Autodesk Inventor part; units mm, degrees
ref_plane "YZ Plane" through (0, 0, 0) normal (1, 0, 0) x (0, 1, 0)
ref_plane "XZ Plane" through (0, 0, 0) normal (0, 1, 0) x (-1, 0, 0)
ref_plane "XY Plane" through (0, 0, 0) normal (0, 0, 1) x (1, 0, 0)
sketch "Skin Scheme" plane through (0, 0, 0) normal (0, 1, 0) x (-1, 0, 0)
  line L0 (464, -84.5) -> (-464, -84.5)
  line L1 (-464, -84.5) -> (-464, 84.5)
  line L2 (-464, 84.5) -> (464, 84.5)
  line L3 (464, 84.5) -> (464, -84.5)
  circle A0 centre (342, -62.5) radius 5
  circle A1 centre (306, -62.5) radius 5
  circle A2 centre (270, -62.5) radius 5
  circle A3 centre (234, -62.5) radius 5
  circle A4 centre (198, -62.5) radius 5
  circle A5 centre (162, -62.5) radius 5
  circle A6 centre (126, -62.5) radius 5
  circle A7 centre (90, -62.5) radius 5
  circle A8 centre (54, -62.5) radius 5
  circle A9 centre (18, -62.5) radius 5
  circle A10 centre (-18, -62.5) radius 5
  circle A11 centre (-54, -62.5) radius 5
  circle A12 centre (-90, -62.5) radius 5
  circle A13 centre (-126, -62.5) radius 5
  circle A14 centre (-162, -62.5) radius 5
  circle A15 centre (-198, -62.5) radius 5
  circle A16 centre (-234, -62.5) radius 5
  circle A17 centre (-270, -62.5) radius 5
  circle A18 centre (342, 62.5) radius 5
  circle A19 centre (306, 62.5) radius 5
  circle A20 centre (270, 62.5) radius 5
  circle A21 centre (234, 62.5) radius 5
  circle A22 centre (198, 62.5) radius 5
  circle A23 centre (162, 62.5) radius 5
  circle A24 centre (126, 62.5) radius 5
  circle A25 centre (90, 62.5) radius 5
  circle A26 centre (54, 62.5) radius 5
  circle A27 centre (18, 62.5) radius 5
  circle A28 centre (-18, 62.5) radius 5
  circle A29 centre (-54, 62.5) radius 5
  circle A30 centre (-90, 62.5) radius 5
  circle A31 centre (-126, 62.5) radius 5
  circle A32 centre (-162, 62.5) radius 5
  circle A33 centre (-198, 62.5) radius 5
  circle A34 centre (-234, 62.5) radius 5
  circle A35 centre (-270, 62.5) radius 5
  circle A36 centre (-306, -62.5) radius 5
  circle A37 centre (-306, 62.5) radius 5
  circle A38 centre (-342, -62.5) radius 5
  circle A39 centre (-342, 62.5) radius 5
  point P0 (0, 0)
  dimension "d0" = 928
  dimension "d1" = 464
  dimension "d2" = 169
  dimension "d3" = 84.5
  dimension "d4" = 10
  dimension "d5" = 122
  dimension "d6" = 22
  dimension "d9" = 36
  dimension "d12" = 125
extrude "Skin Body" add sketch "Skin Scheme" along normal blind 1
sketch "End Cut Outline" plane through (0, 1, 0) normal (0, 1, 0) x (1, 0, 0)
  line L0 (-414, 94.5) -> (-474, 94.5)
  line L1 (-474, 94.5) -> (-474, -94.5)
  line L2 (-474, -94.5) -> (-414, -94.5)
  line L3 (-414, -94.5) -> (-414, 94.5)
  line L4 (464, 84.5) -> (-464, 84.5)
  line L5 (-464, -84.5) -> (464, -84.5)
  line L6 (-464, 84.5) -> (-464, -84.5)
  point P0 (0, 0)
  dimension "d19" = 10
  dimension "d20" = 10
  dimension "d21" = 10
  dimension "d22" = 50
extrude "End Cut" cut sketch "End Cut Outline" along normal through all both and the other way through all
mirror "End Cut Mirror" about plane through (0, 0, 0) normal (1, 0, 0) of "End Cut"
properties part number "Skin NPS 6 Internal" material "Rubber, Silicone"
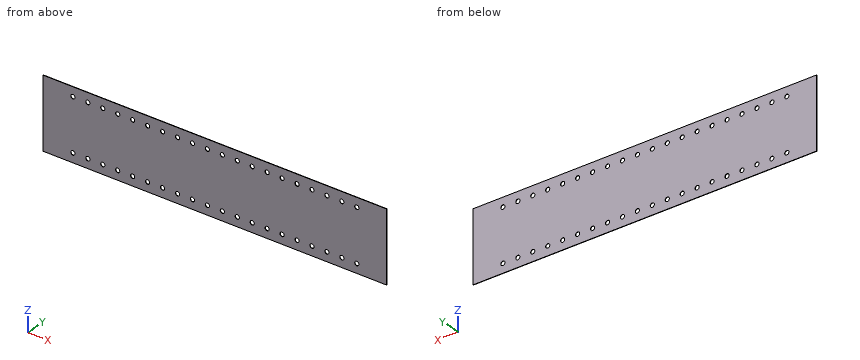
Check sheet for the modelled part. Datum: model origin and axes. Units: mm. Give positions to 0.01 mm unless a question says otherwise; leave off trailing zeros. Answer in a Markdown table with one row per item. Add a question column.
Q1. Gauge pin test, flat end, axial feed: pin 1 Ø11.5 at (x, z) = (-162, -62.5) entering from +Y. Record the tip position at first contact, or that the pin passes through.
Q2. Sectioned sample at A-A, the plane y = 0.6. Count the separate pieces of the cut face and the enclosed holes in it, and give its area (3 significant figures).
Q3. Thickness scan on L1, parallel to Z at x = 18, y = 0.3; L2, parallel to Z at x = 166.5, y = 0.8. Record the ranges inside material, lowest first.
Verdict:
| question | item | result |
|---|---|---|
| 1 | pin 1 | y = 1 |
| 2 | separate pieces | 1 |
| 2 | enclosed holes | 40 |
| 2 | area | 137,000 mm² |
| 3 | L1 | -84.5 to -67.5, -57.5 to 57.5, 67.5 to 84.5 |
| 3 | L2 | -84.5 to -64.68, -60.32 to 60.32, 64.68 to 84.5 |
